```python
from build123d import *

# Parameters (mm, degrees)
SQUARE_TUBE_2X2X188_A500_1_DEPTH = 431.8
CUT_EXTRUDE1_DEPTH               = 436.519276267


with BuildPart() as part:
    # Sketch12 → Square tube 2X2X188 A500(1) (new body)
    with BuildSketch(Plane(origin=(0, 0, 0), x_dir=(0, -1, 0), z_dir=(-1, 0, 0))):
        with BuildLine():
            Line((22.86, -25.4), (-22.86, -25.4))
            ThreePointArc((-22.86, -25.4), (-24.656051224, -24.656051224), (-25.4, -22.86))
            Line((-25.4, -22.86), (-25.4, 22.86))
            ThreePointArc((-25.4, 22.86), (-24.656051224, 24.656051224), (-22.86, 25.4))
            Line((-22.86, 25.4), (22.86, 25.4))
            ThreePointArc((22.86, 25.4), (24.656051224, 24.656051224), (25.4, 22.86))
            Line((25.4, 22.86), (25.4, -22.86))
            ThreePointArc((25.4, -22.86), (24.656051224, -24.656051224), (22.86, -25.4))
        make_face()
        with BuildLine():
            Line((18.56232, 20.6248), (-18.56232, 20.6248))
            ThreePointArc((-18.56232, 20.6248), (-20.020713594, 20.020713594), (-20.6248, 18.56232))
            Line((-20.6248, 18.56232), (-20.6248, -18.56232))
            ThreePointArc((-20.6248, -18.56232), (-20.020713594, -20.020713594), (-18.56232, -20.6248))
            Line((-18.56232, -20.6248), (18.56232, -20.6248))
            ThreePointArc((18.56232, -20.6248), (20.020713594, -20.020713594), (20.6248, -18.56232))
            Line((20.6248, -18.56232), (20.6248, 18.56232))
            ThreePointArc((20.6248, 18.56232), (20.020713594, 20.020713594), (18.56232, 20.6248))
        make_face(mode=Mode.SUBTRACT)
    extrude(amount=SQUARE_TUBE_2X2X188_A500_1_DEPTH)

    # Sketch14 → Cut-Extrude1 (cut, through all)
    with BuildSketch(Plane.XY.offset(25.4)):
        Polygon((-431.8, -25.4), (-431.8, 25.4), (-381, 25.4), align=None)
        Polygon((0, -25.4), (0, 25.4), (-50.8, 25.4), align=None)
    extrude(amount=-CUT_EXTRUDE1_DEPTH, mode=Mode.SUBTRACT)


solid = part.part
```
The model under review builds one solid part; all positions refer to its coordinate system, in mm. A direction names the side the tool comes from. Round coordinates to 2 decimals unless told otherwise and drop trailing zeros. Loops run counter-clockwise (first coordinate to the right, second up) from the corner with the lowest first, then second, coordinate; pieces in that order, holes last. Notation, with made-up numbers: (63, -2) -> (99, -2) arc R18 ccw to (99, 12) -> close; hole circle Ø4 at (-37.75, 50). An arc over 180 degrees is marked (long way). Answer as a JSON object with one key per item and string values. Group by question number.
1) For faces 1 (the face through (-213, -20.625, 0)), 2 (the face through (-213, -25.4, 0)), list the 3-axis set-ups (+Z, -Z, +X, -X, +Y, -Y) from which the entire face can be reached by the end or side of a thin tool; tool diameter is ignored.
2) We need section C-C on x = -126.5. Write out the cut boundary in (y, z), then the cut area to 3 significant figures.
3) Mouldability with a two-part tool opening along Y and no side actions: class faces 3 (the face through (-213, 0, -20.625)), 4 (the face through (-25.8, 0.4, -22.2)), 5 (the face through (-213, 0, -25.4)) as released by +Y, released by -Y, zero draft, split by the parting line, or undercut.
4) We need section B-B on z = 9.5. Write out the cut boundary in (x, y), then the cut area to 3 significant figures.
5) For pin 1 Ø12 at (y, z) = (19.5, -16.5) entering from -X, flat-tipped, find the tip position at first contact; note if it passes through.
6) We need section A-A on y = 8. Write out the cut boundary in (x, z), then the cut area to 3 significant figures.
7) For line 1 (Z direction, x = -202, y = -13); line 2 (Y direction, x = -231, z = 19.5), list the stretches that pass through material, from the lowest coordinate up. Write a range as [from, to].
Result set:
{
 "1": {"face 1": "+X, -X", "face 2": "+Z, -Z, +X, -X, -Y"},
 "2": {"outline": "(-25.4, -22.86) arc R2.54 ccw to (-22.86, -25.4) -> (22.86, -25.4) arc R2.54 ccw to (25.4, -22.86) -> (25.4, 22.86) arc R2.54 ccw to (22.86, 25.4) -> (-22.86, 25.4) arc R2.54 ccw to (-25.4, 22.86) -> close; hole (-20.62, -18.56) arc R2.06 ccw to (-18.56, -20.62) -> (18.56, -20.62) arc R2.06 ccw to (20.62, -18.56) -> (20.62, 18.56) arc R2.06 ccw to (18.56, 20.62) -> (-18.56, 20.62) arc R2.06 ccw to (-20.62, 18.56) -> close", "area": "877 mm²"},
 "3": {"face 3": "undercut", "face 4": "released by +Y", "face 5": "zero draft"},
 "4": {"outline": "(-431.8, -25.4) -> (0, -25.4) -> (-4.78, -20.62) -> (-427.02, -20.62) -> close; (-385.78, 20.62) -> (-46.02, 20.62) -> (-50.8, 25.4) -> (-381, 25.4) -> close", "area": "3,640 mm²"},
 "5": {"pin 1": "x = -391.26"},
 "6": {"outline": "(-398.4, -25.4) -> (-33.4, -25.4) -> (-33.4, -20.62) -> (-398.4, -20.62) -> close; (-398.4, 20.62) -> (-33.4, 20.62) -> (-33.4, 25.4) -> (-398.4, 25.4) -> close", "area": "3,490 mm²"},
 "7": {"line 1": "[-25.4, -20.62], [20.62, 25.4]", "line 2": "[-25.4, -20.4], [20.4, 25.4]"}
}
